```python
from build123d import *

# Parameters (mm, degrees)
BOSS_EXTRUDE1_DEPTH = 5
SKETCH2_R           = 0.75
BOSS_EXTRUDE4_DEPTH = 1


with BuildPart() as part:
    # Sketch1 → Boss-Extrude1 (new body)
    with BuildSketch(Plane(origin=(0, 0, 0), x_dir=(1, 0, 0), z_dir=(0, 1, 0))):
        Polygon((-12.35, 1.5), (-12.35, 7), (12.35, 7), (12.35, 1.5), (12.35, -1.5), (7.35, -1.5), (7.35, -3.5), (14.35, -3.5), (14.35, 9), (-14.35, 9), (-14.35, -3.5), (-7.182955123, -3.5), (-7.182955123, -1.5), (-12.35, -1.5), align=None)
    extrude(amount=BOSS_EXTRUDE1_DEPTH)

    # Sketch2 → Boss-Extrude4 (add)
    with BuildSketch(Plane(origin=(0, 5, 0), x_dir=(1, 0, 0), z_dir=(0, 1, 0))):
        with Locations((0, 8)):
            Circle(SKETCH2_R)
        with Locations((-3, 8)):
            Circle(SKETCH2_R)
        with Locations((3, 8)):
            Circle(SKETCH2_R)
    extrude(amount=BOSS_EXTRUDE4_DEPTH)


solid = part.part
```
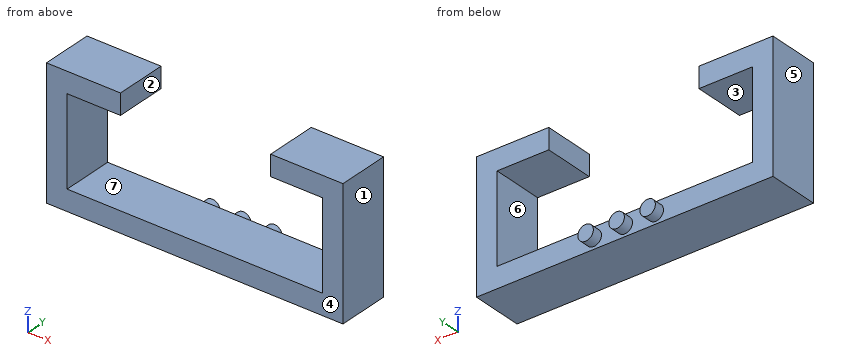
Can you work these out from the model? Positions are in its coordinate system, mm. Face numbers are marked on the shaded views. A direction names the side the tool comes from. Give positions to 0.01 mm unless a question says otherwise; leave off trailing zeros. Loops run counter-clockwise (first coordinate to the right, second up) from the corner with the lowest first, then second, coordinate; pieces in that order, holes last. Notation, with made-up numbers: M -39,85 L -22,85 A11 cw -22,100 Z; hole C 82.5,71 d3. An arc over 180 degrees is marked long. Use CSV: the item, a comma, the result in double quotes. Start each with the question number.
1. If we mould it in two halves opening along X, with no side actions, what happens to the marked faces 4, 5, 6 and 7? For each: released by +X, released by -X, zero draft, split by the parting line, or undercut.
2. Imagine slicing it at C-C, the plane y = 0.7. Write out the boundary of the cut face in (x, z), plus the area to 3 significant figures.
3. Imagine slicing it at B-B, the plane z = -5. Write out the boundary of the cut face in (x, y).
4. For P1, Ø6, axis at x = 10, z = -7, coming from the +Y side, with a flat end and sliding along its axis, tell me the tip position at first contact or that it passes through.
5. On a 3-axis mill with a long thin cutter (end or side, diameter ignored), from which of +Z, -Z, +X, -X, +Y, -Y can I reach the whole of each face in a straight line? I mean the marked faces 1, 2 and 3. Say none if no direction works.
6. If I drill on L1, parallel to X at y = 3.45, z = -5.75; L2, parallel to Z at x = 9.5, y = 2.5; L3, parallel to X at y = 3.25, z = 2.75, over which ranges is the centre line in solid material (lowest first)?
7. Imagine slicing it at A-A, the plane x = -11.25. Write out the boundary of the cut face in (y, z), plus the area to 3 significant figures.
8. Imagine slicing it at D-D, the plane x = 3. Write out the boundary of the cut face in (y, z).
Response values:
1,face 4,"zero draft"
1,face 5,"released by -X"
1,face 6,"undercut"
1,face 7,"undercut"
2,outline,"M -14.35,-9 L 14.35,-9 L 14.35,3.5 L 7.35,3.5 L 7.35,1.5 L 12.35,1.5 L 12.35,-7 L -12.35,-7 L -12.35,1.5 L -7.18,1.5 L -7.18,3.5 L -14.35,3.5 Z"
2,area,"120 mm^2"
3,outline,"M -14.35,0 L -12.35,0 L -12.35,5 L -14.35,5 Z; M 12.35,0 L 14.35,0 L 14.35,5 L 12.35,5 Z"
4,P1,"y = 5"
5,face 1,"+Z, -Z, +X, +Y, -Y"
5,face 2,"+Z, +Y, -Y"
5,face 3,"+Y, -Y"
6,L1,"-14.35 to -12.35, 12.35 to 14.35"
6,L2,"-9 to -7, 1.5 to 3.5"
6,L3,"-14.35 to -7.18, 7.35 to 14.35"
7,outline,"M 0,-9 L 5,-9 L 5,-7 L 0,-7 Z; M 0,1.5 L 5,1.5 L 5,3.5 L 0,3.5 Z"
7,area,"20.0 mm^2"
8,outline,"M 0,-9 L 5,-9 L 5,-8.75 L 6,-8.75 L 6,-7.25 L 5,-7.25 L 5,-7 L 0,-7 Z"
